Input: dimensioned drawing with shaded views. Units: mm. Origin: part minimum x, y, z. Round coordinates to 2 decimals unless told otherwise and drop trailing zeros. Loops run counter-clockwise (first coordinate to the right, second up) from the corner with the lowest first, then second, coordinate; pieces in that order, holes last. Notation, with made-up numbers: M 42,55.25 L 90,55.25 A21 cw 90,66.25 Z; hole C -19.75,68.5 d5. An arc over 180 degrees is marked long. Return JSON: item names as keys, results as strings.
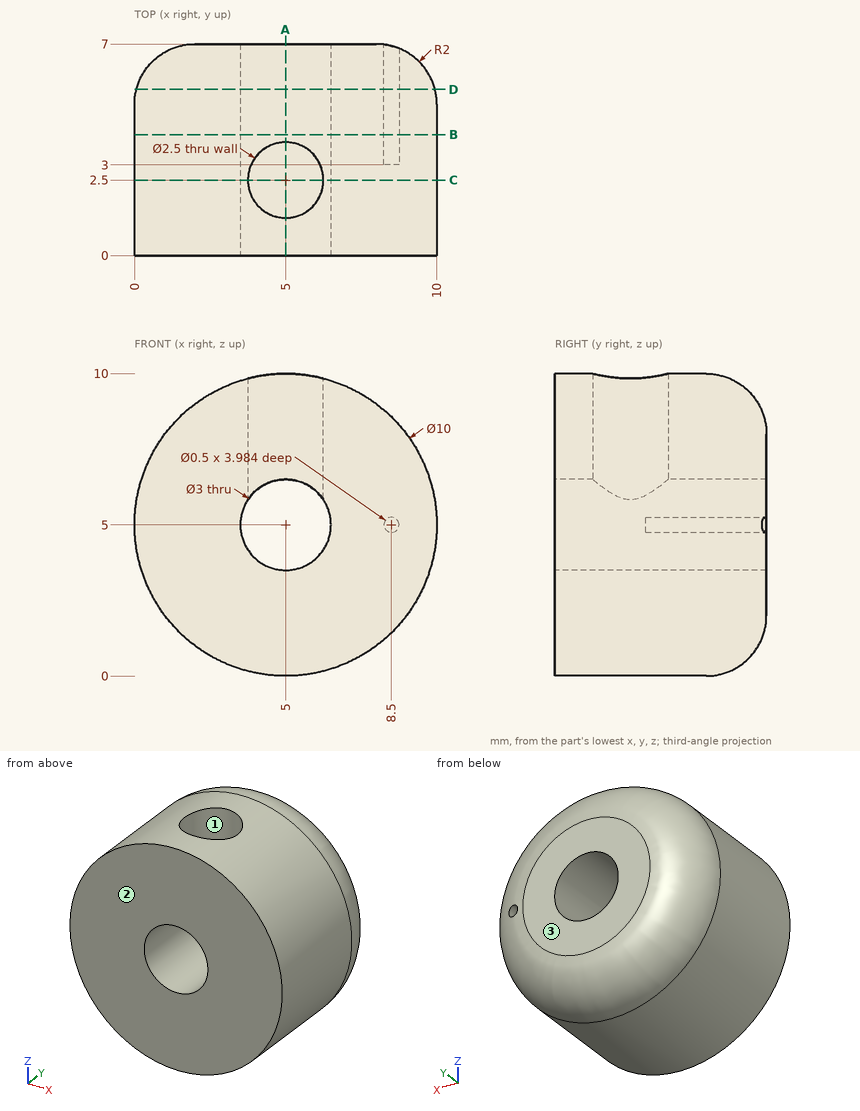
Q1. Material intervals for L1, parallel to Y at x = 5, z = 6.75; L2, parallel to Z at x = 9, y = 4; L3, parallel to Z at x = 5, y = 4.25, sorted ascending.
Determined:
{"L1": "y = 0 to 1.25, 3.75 to 7", "L2": "z = 2 to 8", "L3": "z = 0 to 3.5, 6.5 to 10"}
Q2. Section query B-B (y = 4). Output: boundary loops of the cut face in (x, z).
Determined:
{"outline": "C 5,5 d10; hole C 5,5 d3; hole C 8.5,5 d0.5"}
Q3. Section query C-C (y = 2.5). Output: boundary loops of the cut face in (x, z).
Determined:
{"outline": "M 3.75,5.83 L 3.75,9.84 A5 ccw long 6.25,9.84 L 6.25,5.83 A1.5 cw long Z"}
Q4. Pull-direction query (Y, two-part tool) for the marked faces 1, 2 and 3; classes: pulls with the +Y half, pulls with the -Y half, needs draft (parallel to the pull), parting line crosses it, or undercut.
Determined:
{"face 1": "undercut", "face 2": "pulls with the -Y half", "face 3": "pulls with the +Y half"}
Q5. Section query A-A (x = 5). State how many separate pieces and enclosed holes the cut face has.
Determined:
{"separate pieces": "3", "enclosed holes": "0"}
Q6. Pin query (flat end, axial travel): pin 1 (2 mm diameter, centred on y = 4, z = 2, fed in from -X); pin 2 (1 mm diameter, centred on y = 3, z = 6.5, fed in from +X). Return the tip coordinate at first contact, or that it passes through.
Determined:
{"pin 1": "stops at x = 0.42", "pin 2": "stops at x = 9.9"}
Q7. Section query D-D (y = 5.5). Output: boundary loops of the cut face in (x, z).
Determined:
{"outline": "C 5,5 d9.87; hole C 5,5 d3; hole C 8.5,5 d0.5"}
